```python
from build123d import *

# Parameters (mm, degrees)
F0_W          = 1800
F0_H          = 1000
F1_DEPTH      = 10
F1_DEPTH_BACK = 20
F1_TAPER_BACK = 60
F3_D          = 7
F3_DEPTH      = 20
F3_TIP        = 2.1030121666


with BuildPart() as f1:
    # F0 (on Top) → F1 (new body, two sides)
    with BuildSketch(Plane.XY) as f1_sk:
        Rectangle(F0_W, F0_H)
    extrude(amount=F1_DEPTH)
    extrude(f1_sk.sketch, amount=-F1_DEPTH_BACK, taper=F1_TAPER_BACK)

    # F3
    with Locations(Plane(origin=(0, 0, -20), x_dir=(1, 0, 0), z_dir=(0, 0, -1))):
        with Locations((800, -345), (800, -115), (800, 115), (800, 345), (750, 400), (450, 400), (150, 400), (-150, 400), (-450, 400), (-750, 400), (450, -400), (150, -400), (-150, -400), (-150, -400), (-800, -345), (-800, -115), (-800, 115), (-450, -400), (-750, -400), (750, -400), (-800, 345), (-265, 345), (-265, 115), (-265, -115), (-265, -345), (265, -345), (265, -345), (265, -115), (265, 345), (265, 115)):
            Hole(F3_D / 2, depth=F3_DEPTH)
            with Locations((0, 0, -(F3_DEPTH + F3_TIP / 2))):  # 118° drill point
                Cone(0, F3_D / 2, F3_TIP, mode=Mode.SUBTRACT)


solid = f1.part
```
Model file for the job. Use its own axes, mm. Give positions to 0.01 mm unless a question says otherwise; leave off trailing zeros. One line per question, with ' | ' between items. Start each with the question number.
(1) Wall check: line 1 along Y through (x, z) = (-150, -15); line 2 along Y through (x, z) = (-265, -4.5); line 3 along X through (y, z) = (-115, -8). Give the ranges that are in metal, low to high. Write a range as from..to.
(2) Slice it at A-A on z = -5.5. Give the number of separate pieces and of enclosed holes in the cut face, plus the area to 3 significant figures.
(3) Pin check, flat tips, straight feed: P1, Ø6.5, axis at x = -800, y = 115, coming from the -Z side; P2, Ø5.5, axis at x = 800, y = 115, coming from the -Z side; P3, Ø4, axis at x = 800, y = -345, coming from the -Z side. Stop position of each tip, or through.
Results below:
1) line 1: -474.02..-403.5, -396.5..396.5, 403.5..474.02 | line 2: -492.21..-348.5, -341.5..-118.5, -111.5..111.5, 118.5..341.5, 348.5..492.21 | line 3: -886.14..-803.5, -796.5..-268.5, -261.5..261.5, 268.5..796.5, 803.5..886.14
2) separate pieces: 1 | enclosed holes: 28 | area: 1,750,000 mm^2
3) P1: z = 0.15 | P2: z = 0.45 | P3: z = 0.9
